Work out the finished part from the listing and answer in its coordinate system (mm). A direction names the side the tool comes from. Coordinates: 2 decimals unless noted, no trailing zeros. Write each loop counter-clockwise with the first axis right and the second up, starting at its lowest first coordinate (ties: lowest second). Pieces come first, ordered by that corner, then holes. Notation, with made-up numbers: (79, -26) - (86, -26) arc R31 cw to (86, 5) - close; hole circle Ø2 at (-10.5, 2.5). An arc over 180 degrees is marked (long way). One line per item, written item: value.
```python
from build123d import *

# Parameters (mm, degrees)
SKETCH2_R           = 1.6
BOSS_EXTRUDE1_DEPTH = 3
CUT_EXTRUDE1_DEPTH  = 85.905830189
BOSS_EXTRUDE2_DEPTH = 3
SHELL1_T            = -2
BOSS_EXTRUDE4_DEPTH = 3


with BuildPart() as part:
    # Sketch2 → Boss-Extrude1 (new body)
    with BuildSketch(Plane(origin=(0, 0, 0), x_dir=(1, 0, 0), z_dir=(0, 1, 0))):
        Polygon((-24.852813742, 60), (-60, 24.852813742), (-60, -24.852813742), (-24.852813742, -60), (24.852813742, -60), (60, -24.852813742), (60, 24.852813742), (24.852813742, 60), align=None)
        with Locations(Location((-38.890872965, -38.890872965, 0), (0, 0, 270))):
            Circle(SKETCH2_R, mode=Mode.SUBTRACT)
        with Locations(Location((38.890872965, 38.890872965, 0), (0, 0, 270))):
            Circle(SKETCH2_R, mode=Mode.SUBTRACT)
        with Locations(Location((0, -55, 0), (0, 0, 270))):
            Circle(SKETCH2_R, mode=Mode.SUBTRACT)
        with Locations(Location((0, 55, 0), (0, 0, 270))):
            Circle(SKETCH2_R, mode=Mode.SUBTRACT)
        with Locations(Location((38.890872965, -38.890872965, 0), (0, 0, 270))):
            Circle(SKETCH2_R, mode=Mode.SUBTRACT)
        with Locations(Location((-38.890872965, 38.890872965, 0), (0, 0, 270))):
            Circle(SKETCH2_R, mode=Mode.SUBTRACT)
        with Locations(Location((55, 0, 0), (0, 0, 270))):
            Circle(SKETCH2_R, mode=Mode.SUBTRACT)
        with Locations(Location((-55, 0, 0), (0, 0, 270))):
            Circle(SKETCH2_R, mode=Mode.SUBTRACT)
    extrude(amount=BOSS_EXTRUDE1_DEPTH)

    # Sketch3 → Cut-Extrude1 (cut, through all)
    with BuildSketch(Plane(origin=(0, 3, 0), x_dir=(1, 0, 0), z_dir=(0, 1, 0))):
        Polygon((20.710678119, 50), (-20.710678119, 50), (-50, 20.710678119), (-50, -20.710678119), (-20.710678119, -50), (20.710678119, -50), (50, -20.710678119), (50, 20.710678119), align=None)
    extrude(amount=-CUT_EXTRUDE1_DEPTH, mode=Mode.SUBTRACT)



with BuildPart() as body_2:
    # Sketch4 → Boss-Extrude2 (new body)
    with BuildSketch(Plane(origin=(0, 18, 0), x_dir=(1, 0, 0), z_dir=(0, 1, 0))):
        Polygon((-40, 16.568542495), (-40, -16.568542495), (-16.568542495, -40), (16.568542495, -40), (40, -16.568542495), (40, 16.568542495), (16.568542495, 40), (-16.568542495, 40), align=None)
    extrude(amount=BOSS_EXTRUDE2_DEPTH)

    # Sketch3<3> → section 0 of loft1
    with BuildSketch(Plane(origin=(0, 3, 0), x_dir=(1, 0, 0), z_dir=(0, 1, 0)), mode=Mode.PRIVATE) as loft1_s0:
        with BuildLine():
            Line((-50, 20.710678119), (-50, -20.710678119))
            Line((-50, -20.710678119), (-20.710678119, -50))
            Line((-20.710678119, -50), (20.710678119, -50))
            Line((20.710678119, -50), (50, -20.710678119))
            Line((50, -20.710678119), (50, 20.710678119))
            Line((50, 20.710678119), (20.710678119, 50))
            Line((20.710678119, 50), (-20.710678119, 50))
            Line((-20.710678119, 50), (-50, 20.710678119))
        make_face()
    # loft up to a face of the part (loft1)
    loft([loft1_s0.sketch, body_2.faces().sort_by_distance((0, 21, 0))[0]])

    # Shell1
    shell1_openings = [body_2.faces().sort_by_distance(p)[0] for p in [
        (0, 3, 0),
    ]]
    offset(amount=SHELL1_T, openings=shell1_openings, kind=Kind.INTERSECTION)


with BuildPart() as part_1:
    add(part.part)

    add(body_2.part)  # Boss-Extrude4 merges body 2
    # Sketch5 → Boss-Extrude4 (add)
    with BuildSketch(Plane.XZ.offset(-3)):
        Polygon((-50, 20.710678119), (-50, -20.710678119), (-20.710678119, -50), (20.710678119, -50), (50, -20.710678119), (50, 20.710678119), (20.710678119, 50), (-20.710678119, 50), align=None)
        Polygon((-47.712082191, 19.762991533), (-47.712082191, -19.762991533), (-19.762991533, -47.712082191), (19.762991533, -47.712082191), (47.712082191, -19.762991533), (47.712082191, 19.762991533), (19.762991533, 47.712082191), (-19.762991533, 47.712082191), align=None, mode=Mode.SUBTRACT)
    extrude(amount=BOSS_EXTRUDE4_DEPTH)


solid = part_1.part
```
Item 1: Section B-B, the plane z = -55 is taken. Determine the outline of the cut face in (x, y), then the cut area to 3 significant figures.
Evaluation:
outline: (-29.85, 0) - (-1.6, 0) - (-1.6, 3) - (-29.85, 3) - close; (1.6, 0) - (29.85, 0) - (29.85, 3) - (1.6, 3) - close
area: 170 mm2
Item 2: Given pin 1 (12 mm diameter, centred on x = -39.5, y = 2.5, fed in from +Z); pin 2 (1.5 mm diameter, centred on x = -9.5, y = 10.5, fed in from -Z); pin 3 (4 mm diameter, centred on x = 55, z = 0, fed in from +Y), each flat-ended and moving along its own axis, determine where each tip first touches the part or whether it passes through.
Evaluation:
pin 1: stops at z = 51.35
pin 2: stops at z = -46.25
pin 3: stops at y = 3
Item 3: Determine the mould class of faces 4 (the face through (-42.18, 1.48, -42.67)), 5 (the face through (0.277, 11.112, -43.205)), 6 (the face through (42.67, 1.48, -42.18)) for opening direction X: +X half, -X half, draft (parallel to the pull), parting line (faces both ways), or undercut.
Evaluation:
face 4: -X half
face 5: undercut
face 6: +X half
Item 4: Consider probe 1 along X at (y, z) = (0.65, 0); probe 2 along Z at (x, y) = (13.5, 1); probe 3 along Y at (x, z) = (22.5, 28). Determine where each line is inside the solid, lowest interval first.
Evaluation:
probe 1: x = -60 to -56.6, -53.4 to -47.71, 47.71 to 53.4, 56.6 to 60
probe 2: z = -60 to -47.71, 47.71 to 60
probe 3: y = 19 to 21
Item 5: Section C-C, the plane x = 0 is taken. Give the number of separate pieces and of enclosed holes in the cut face, then the cut area to 3 significant figures.
Evaluation:
separate pieces: 3
enclosed holes: 0
area: 290 mm2
Item 6: Which of the six approach directions +Z, -Z, +X, -X, +Y, -Y give full straight-line access (tool end or side, diameter ignored) to faces 1 (the face through (-43.205, 11.112, -0.277)), 2 (the face through (0.481, 1.479, -53.474)), 3 (the face through (-31, 3, 40))?
Evaluation:
face 1: -Y
face 2: +Y, -Y
face 3: +Y
Item 7: Section A-A, the plane x = -55 is taken. Determine the outline of the cut face in (y, z), then the cut area to 3 significant figures.
Evaluation:
outline: (0, -29.85) - (3, -29.85) - (3, -1.6) - (0, -1.6) - close; (0, 1.6) - (3, 1.6) - (3, 29.85) - (0, 29.85) - close
area: 170 mm2
